Build history of the part. All positions in model axes, mm. A direction names the side the tool comes from. Round coordinates to 2 decimals unless told otherwise and drop trailing zeros. Write each loop counter-clockwise with the first axis right and the second up, starting at its lowest first coordinate (ties: lowest second). Pieces come first, ordered by that corner, then holes. Notation, with made-up numbers: (80.5, 82) -> (89.5, 82) arc R16 cw to (89.5, 96) -> close; hole circle Ø11 at (45, -33.75). An arc over 180 degrees is marked (long way). Answer in a Markdown table with one row per item.
```python
from build123d import *

# Parameters (mm, degrees)
SKETCH3_W             = 35.921024484
SKETCH3_H             = 35.921024484
BOSS_EXTRUDE2_DEPTH   = 12.7
BOSS_EXTRUDE3_DEPTH   = 25.4
F_8_CLEARANCE_HOLE1_D = 4.9149
F_8_CLEARANCE_HOLE2_D = 4.9149
SKETCH10_R            = 3.937
CUT_EXTRUDE1_DEPTH    = 6.35
FILLET1_R             = 2.54


with BuildPart() as part:
    # Sketch3 → Boss-Extrude2 (new body)
    with BuildSketch(Plane(origin=(0, 0, 0), x_dir=(1, 0, 0), z_dir=(0, 1, 0))):
        with Locations((17.960512242, -17.960512242)):
            Rectangle(SKETCH3_W, SKETCH3_H)
    extrude(amount=BOSS_EXTRUDE2_DEPTH)

    # Sketch4 → Boss-Extrude3 (add, symmetric)
    with BuildSketch(Plane(origin=(0, 0, 0), x_dir=(0.7071067811865476, 0, 0.7071067811865475), z_dir=(-0.7071067811865475, 0, 0.7071067811865476))):
        Polygon((25.4, 12.7), (-25.4, 12.7), (-50.8, 12.7), (-50.8, 0), (0, 0), (25.4, 0), align=None)
    extrude(amount=BOSS_EXTRUDE3_DEPTH, both=True)

    # #8 Clearance Hole1 (through all)
    with Locations(Plane(origin=(0, 0, 0), x_dir=(-1, 0, 0), z_dir=(0, -1, 0))):
        with Locations((-29.571024484, -29.571024484), (-4.171024484, -4.171024484), (-29.571024484, -4.171024484), (-4.171024484, -29.571024484)):
            Hole(F_8_CLEARANCE_HOLE1_D / 2)

    # #8 Clearance Hole2 (through all)
    with Locations(Plane(origin=(0, 12.7, 0), x_dir=(1, 0, 0), z_dir=(0, 1, 0))):
        with Locations((-40.855979707, 15.459815396), (-15.459815396, 40.855979707)):
            Hole(F_8_CLEARANCE_HOLE2_D / 2)

    # Sketch10 → Cut-Extrude1 (cut)
    with BuildSketch(Plane.XZ):
        with Locations(Location((-40.855979707, -15.459815396, 0), (0, 0, 270))):
            Circle(SKETCH10_R)
        with Locations(Location((-15.459815396, -40.855979707, 0), (0, 0, 270))):
            Circle(SKETCH10_R)
    extrude(amount=-CUT_EXTRUDE1_DEPTH, mode=Mode.SUBTRACT)

    # Fillet1
    fillet1_edges = [part.edges().sort_by_distance(p)[0] for p in [
        (-17.960512242, 6.35, -53.881536726),
        (-53.881536726, 6.35, -17.960512242),
        (35.921024484, 6.35, 0),
        (35.921024484, 6.35, 35.921024484),
        (0, 6.35, 35.921024484),
    ]]
    fillet(fillet1_edges, radius=FILLET1_R)


solid = part.part
```
Q1. Saw through at B-B on z = 23. Write the cut outline in (x, y), plus the area to 3 significant figures.
A:
| item | result |
|---|---|
| outline | (-12.92, 0) -> (35.92, 0) -> (35.92, 12.7) -> (-12.92, 12.7) -> close |
| area | 620 mm² |
Q2. Saw through at D-D on x = 10. Write the cut outline in (y, z), plus the area to 3 significant figures.
A:
| item | result |
|---|---|
| outline | (0, -25.92) -> (12.7, -25.92) -> (12.7, 35.92) -> (0, 35.92) -> close |
| area | 785 mm² |
Q3. Drop flat-ended pins along their axis: P1, Ø1, axis at y = 9.5, z = -12.5, coming from the -X side; P2, Ø1.5, axis at x = -7, y = 8, coming from the +Z side; P3, Ø5.5, axis at x = -15.46, z = -40.86, coming from the -Y side. Give the stop position or say it passes through.
A:
| item | result |
|---|---|
| P1 | x = -48.92 |
| P2 | z = 29.67 |
| P3 | y = 6.35 |
Q4. Two-plate mould, pull along Z, no slides. Class faces 1 (the flat face through (-1, 0, -1)), 2 (the cylindrical face through (-52.83, 6.26, -17.93)), 3 (the cylindrical face through (3.851, 6.439, 27.134)), 4 (the cylindrical face through (-14.927, 9.481, -38.457)): released by +Z, released by -Z, zero draft, split by the parting line, or undercut.
A:
| item | result |
|---|---|
| face 1 | zero draft |
| face 2 | split by the parting line |
| face 3 | undercut |
| face 4 | undercut |
Q5. Which spindle directions (+Z, -Z, +X, -X, +Y, -Y) get a long thin tool onto all of the face, cutting with end or side? Do faces 5 (the flat face through (-42, 6.35, -18)), 6 (the cylindrical face through (31.915, 6.439, 3.433)). Say none if no direction does.
A:
| item | result |
|---|---|
| face 5 | -Y |
| face 6 | +Y, -Y |
Q6. Wall check: line 1 (X direction, y = 9.5, z = 2); line 2 (X direction, y = 12, z = 28); line 3 (X direction, y = 3.75, z = -12). Give the ranges that are in metal, low to high. Write a range as [from, to].
A:
| item | result |
|---|---|
| line 1 | [-33.92, 3.02], [5.32, 28.42], [30.72, 35.92] |
| line 2 | [-7.92, 2.28], [6.06, 27.68], [31.46, 35.92] |
| line 3 | [-47.92, -42.73], [-38.98, 23.92] |
Q7. Saw through at C-C on y = 10. Write the cut outline in (x, z), plus the area to 3 significant figures.
A:
| item | result |
|---|---|
| outline | (-52.09, -19.76) -> (-19.76, -52.09) arc R2.54 ccw to (-16.16, -52.09) -> (35.18, -0.74) arc R2.54 ccw to (35.92, 1.05) -> (35.92, 33.38) arc R2.54 ccw to (33.38, 35.92) -> (1.05, 35.92) arc R2.54 ccw to (-0.74, 35.18) -> (-52.09, -16.16) arc R2.54 ccw to start; hole circle Ø4.91 at (-40.86, -15.46); hole circle Ø4.91 at (-15.46, -40.86); hole circle Ø4.91 at (4.17, 4.17); hole circle Ø4.91 at (4.17, 29.57); hole circle Ø4.91 at (29.57, 4.17); hole circle Ø4.91 at (29.57, 29.57) |
| area | 4,400 mm² |
Q8. Saw through at A-A on y = 3. Write the cut outline in (x, z), plus the area to 3 significant figures.
A:
| item | result |
|---|---|
| outline | (-52.09, -19.76) -> (-19.76, -52.09) arc R2.54 ccw to (-16.16, -52.09) -> (35.18, -0.74) arc R2.54 ccw to (35.92, 1.05) -> (35.92, 33.38) arc R2.54 ccw to (33.38, 35.92) -> (1.05, 35.92) arc R2.54 ccw to (-0.74, 35.18) -> (-52.09, -16.16) arc R2.54 ccw to start; hole circle Ø7.87 at (-40.86, -15.46); hole circle Ø7.87 at (-15.46, -40.86); hole circle Ø4.91 at (4.17, 4.17); hole circle Ø4.91 at (4.17, 29.57); hole circle Ø4.91 at (29.57, 4.17); hole circle Ø4.91 at (29.57, 29.57) |
| area | 4,340 mm² |
